from build123d import *

# Parameters (mm, degrees)
CHAMFER_1_SIZE     = 0.5
HOLE_WIZARD_M3_2_D = 2.5


with BuildPart() as part:
    # 草图1 → 旋转1 (revolve)
    with BuildSketch(Plane.XY, mode=Mode.PRIVATE) as revolve_1_sk:
        Polygon((5, 0), (5, 20), (2.5, 20), (2.5, 30), (7.5, 30), (7.5, 0), align=None)
    revolve(revolve_1_sk.sketch.rotate(Axis((0, 0, 0), (0, 1, 0)), 90), axis=Axis((0, 0, 0), (0, 1, 0)))

    # 倒角1
    chamfer_1_edges = [part.edges().sort_by_distance(p)[0] for p in [
        (0, 0, 7.5),
        (0, 30, 7.5),
        (0, 30, 2.5),
        (0, 0, 5),
    ]]
    chamfer(chamfer_1_edges, length=CHAMFER_1_SIZE)

    # M3 螺纹孔2 (through all)
    with Locations(Plane.XY.offset(7.5)):
        with Locations((0, 26), (0, 9)):
            Hole(HOLE_WIZARD_M3_2_D / 2)


solid = part.part
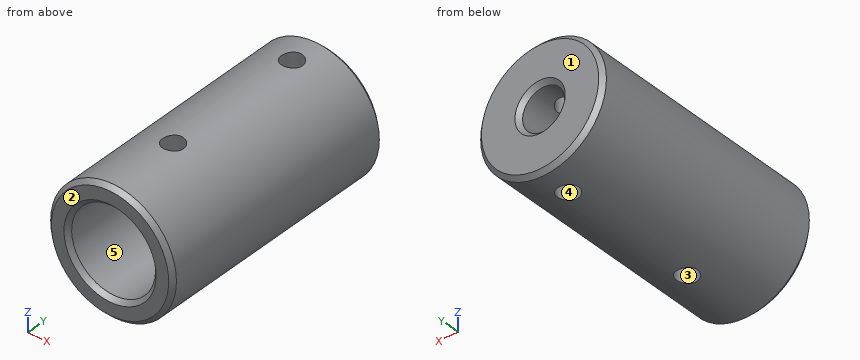
Geometry check sheet. Reference: the model listing, model coordinates, mm. Face numbers are marked on the shaded views. A direction names the side the tool comes from. Round coordinates to 2 decimals unless told otherwise and drop trailing zeros. Loops run counter-clockwise (first coordinate to the right, second up) from the corner with the lowest first, then second, coordinate; pieces in that order, holes last.
Item 1: Cross-section at B-B on y = 9. Record the boundary of the cut face in (x, z), then the cut area to 3 significant figures.
Item 2: Cross-section at D-D on y = 26. Record the boundary of the cut face in (x, z), then the cut area to 3 significant figures.
Item 3: Gauge pin test, flat ends, axial feed: pin 1 (2 mm diameter, centred on x = 3.5, y = 10.5, fed in from +Z); pin 2 (8 mm diameter, centred on x = -1, z = -1, fed in from -Y); pin 3 (2 mm diameter, centred on x = 0, y = 26, fed in from +Z); pin 4 (8 mm diameter, centred on x = 0, z = 0, fed in from -Y). Record the tip position at first contact, or that the pin passes through.
Item 4: Mould release check, pull along Y, two halves, no side actions. Record for the marked faces 1, 2 and 3: pulls with the +Y half, pulls with the -Y half, needs draft (parallel to the pull), parting line crosses it, or undercut.
Item 5: Cross-section at A-A on z = 0. Record the boundary of the cut face in (x, y), then the cut area to 3 significant figures.
Item 6: Cross-section at C-C on x = 0. Count the separate pieces of the cut face and the enclosed holes in it, then the cut area to 4 significant figures.
Item 7: Access from +Z, -Z, +X, -X, +Y, -Y to the whole of each face (thin tool, end or side, straight path). Record for the marked faces 4 and 5.
Item 8: Thickness scan on line 1 (X direction, y = 10.5, z = 0); line 2 (X direction, y = 27.75, z = 0); line 3 (Y direction, x = -3.5, z = 0.25). Record the ranges inside material, lowest first.
Answer sheet:
1. outline: (-1.25, -7.4) - (-1.25, -4.84) arc R5 cw to (-1.25, 4.84) - (-1.25, 7.4) arc R7.5 ccw to start; (1.25, -7.4) arc R7.5 ccw to (1.25, 7.4) - (1.25, 4.84) arc R5 cw to (1.25, -4.84) - close
1. area: 85.6 mm2
2. outline: (-1.25, -7.4) - (-1.25, -2.17) arc R2.5 cw to (-1.25, 2.17) - (-1.25, 7.4) arc R7.5 ccw to start; (1.25, -7.4) arc R7.5 ccw to (1.25, 7.4) - (1.25, 2.17) arc R2.5 cw to (1.25, -2.17) - close
2. area: 132 mm2
3. pin 1: stops at z = 7.07
3. pin 2: stops at y = 0.09
3. pin 3: passes through
3. pin 4: stops at y = 20
4. face 1: pulls with the +Y half
4. face 2: pulls with the -Y half
4. face 3: undercut
5. outline: (-7.5, 0.5) - (-7, 0) - (-5.5, 0) - (-5, 0.5) - (-5, 20) - (-2.5, 20) - (-2.5, 29.5) - (-3, 30) - (-7, 30) - (-7.5, 29.5) - close; (2.5, 20) - (5, 20) - (5, 0.5) - (5.5, 0) - (7, 0) - (7.5, 0.5) - (7.5, 29.5) - (7, 30) - (3, 30) - (2.5, 29.5) - close
5. area: 199 mm2
6. separate pieces: 6
6. enclosed holes: 0
6. area: 161.5 mm2
7. face 4: +Z, -Z
7. face 5: -Y
8. line 1: x = -7.5 to -5, 5 to 7.5
8. line 2: x = -7.5 to -2.5, 2.5 to 7.5
8. line 3: y = 20 to 30
